Part model, mm, in its own coordinate system. Face numbers are marked on the shaded views. A direction names the side the tool comes from. Give positions to 0.01 mm unless a question says otherwise; leave off trailing zeros. Write each loop counter-clockwise with the first axis right and the second up, starting at its lowest first coordinate (ties: lowest second). Pieces come first, ordered by that corner, then holes. Notation, with made-up numbers: (66, 20.5) - (116, 20.5) arc R16 ccw to (116, 47.5) - close; hole circle Ø7 at (59.5, -25.75). An arc over 180 degrees is marked (long way). Answer in a Markdown table with one row per item. Add a question column.
1. Band-saw the part on C-C on y = -55.88. Write the cut outline in (x, z), plus the area to 3 significant figures.
2. Band-saw the part on A-A on x = 0. Write the cut outline in (y, z).
3. Which spindle directions (+Z, -Z, +X, -X, +Y, -Y) get a long thin tool onto all of the face, cutting with end or side? Do the marked faces 4, 5 and 6. Say none if no direction does.
4. Band-saw the part on B-B on z = 2. Write the cut outline in (x, y).
5. Band-saw the part on D-D on z = 33.5. Write the cut outline in (x, y), plus the area to 3 significant figures.
6. Pull direction X, two halves, no side cores. Call the marked faces 1, 2 and 3: released by +X, released by -X, zero draft, split by the parting line, or undercut.
7. Drop flat-ended pins along their axis: pin 1 Ø2.5 at (x, z) = (0, 9.5) entering from -Y; pin 2 Ø8.5 at (x, z) = (10.5, 40.5) entering from -Y; pin 3 Ø12 at (x, y) = (1.5, 35.5) entering from +Z. Give the stop position or say it passes through.
8. Probe line 1 along Y through (x, z) = (0, -7); line 2 along Y through (x, z) = (0, -3.5); line 3 along X through (y, z) = (-83.5, 12). List the from-to ranges inside material, lowest first.
```python
from build123d import *

# Parameters (mm, degrees)
F0_R           = 10.16
F1_DEPTH       = 38.1
F3_START       = 7.62
F3_DEPTH       = 27.941
F4_D           = 15.24
F4_CBORE_D     = 40.64
F4_CBORE_DEPTH = 10.16
F2_W           = 5.08
F2_H           = 76.2
F5_DEPTH       = 10.16
F6_R           = 10.16


with BuildPart() as f1:
    # F0 (on Right) → F1 (new body, symmetric)
    with BuildSketch(Plane.YZ):
        Polygon((-17.78, 15.24), (-93.98, 15.24), (-93.98, -20.32), (17.78, -20.32), (53.34, 15.24), (53.34, 50.8), (17.78, 50.8), align=None)
        Circle(F0_R, mode=Mode.SUBTRACT)
    extrude(amount=F1_DEPTH, both=True)

    # F2 (on face) → F3 (cut)
    with BuildSketch(Plane.XY.offset(15.24).offset(F3_START)):
        with BuildLine():
            Line((22.86, 43.18), (-22.86, 43.18))
            ThreePointArc((-22.86, 43.18), (-30.48, 35.56), (-22.86, 27.94))
            Line((-22.86, 27.94), (22.86, 27.94))
            ThreePointArc((22.86, 27.94), (30.48, 35.56), (22.86, 43.18))
        make_face()
    extrude(amount=F3_DEPTH, mode=Mode.SUBTRACT)

    # F4 (through all)
    with Locations(Plane.XY.offset(15.24)):
        with Locations((0, -55.88)):
            CounterBoreHole(F4_D / 2, F4_CBORE_D / 2, F4_CBORE_DEPTH)

    # F2 (on face) → F5 (cut)
    with BuildSketch(Plane.XY.offset(15.24)):
        with Locations((0, -55.88)):
            Rectangle(F2_W, F2_H)
    extrude(amount=-F5_DEPTH, mode=Mode.SUBTRACT)

    # F6
    f6_edges = [f1.edges().sort_by_distance(p)[0] for p in [
        (38.1, -93.98, -2.54),
        (-38.1, -93.98, -2.54),
        (38.1, 53.34, 33.02),
        (-38.1, 53.34, 33.02),
    ]]
    fillet(f6_edges, radius=F6_R)


solid = f1.part
```
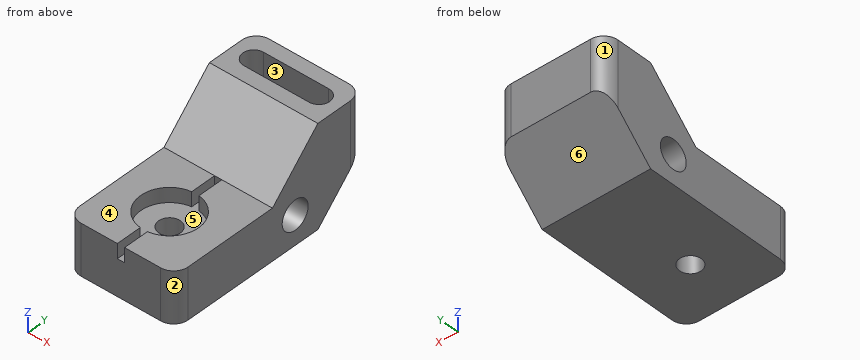
Values:
| question | item | result |
|---|---|---|
| 1 | outline | (-38.1, -20.32) - (-7.62, -20.32) - (-7.62, 5.08) - (-20.32, 5.08) - (-20.32, 15.24) - (-38.1, 15.24) - close; (7.62, -20.32) - (38.1, -20.32) - (38.1, 15.24) - (20.32, 15.24) - (20.32, 5.08) - (7.62, 5.08) - close |
| 1 | area | 1,910 mm² |
| 2 | outline | (-93.98, -20.32) - (-63.5, -20.32) - (-63.5, 5.08) - (-93.98, 5.08) - close; (-48.26, -20.32) - (17.78, -20.32) - (53.34, 15.24) - (53.34, 50.8) - (43.18, 50.8) - (43.18, 22.86) - (27.94, 22.86) - (27.94, 50.8) - (17.78, 50.8) - (-17.78, 15.24) - (-17.78, 5.08) - (-48.26, 5.08) - close; hole circle Ø20.32 at (0, 0) |
| 3 | face 4 | +Z, +X, -X, -Y |
| 3 | face 5 | +Z |
| 3 | face 6 | -Z, +X, -X, +Y |
| 4 | outline | (-38.1, -83.82) arc R10.16 ccw to (-27.94, -93.98) - (27.94, -93.98) arc R10.16 ccw to (38.1, -83.82) - (38.1, -9.96) - (-38.1, -9.96) - close; (-38.1, 9.96) - (38.1, 9.96) - (38.1, 40.1) - (-38.1, 40.1) - close; hole circle Ø15.24 at (0, -55.88) |
| 5 | outline | (-38.1, 0.48) - (38.1, 0.48) - (38.1, 43.18) arc R10.16 ccw to (27.94, 53.34) - (-27.94, 53.34) arc R10.16 ccw to (-38.1, 43.18) - close; hole (-22.86, 27.94) - (22.86, 27.94) arc R7.62 ccw to (22.86, 43.18) - (-22.86, 43.18) arc R7.62 ccw to start |
| 5 | area | 3,100 mm² |
| 6 | face 1 | released by -X |
| 6 | face 2 | released by +X |
| 6 | face 3 | undercut |
| 7 | pin 1 | stops at y = -17.78 |
| 7 | pin 2 | stops at y = 3.23 |
| 7 | pin 3 | stops at z = 22.86 |
| 8 | line 1 | y = -93.98 to -63.5, -48.26 to -7.36, 7.36 to 31.1 |
| 8 | line 2 | y = -93.98 to -63.5, -48.26 to -9.54, 9.54 to 34.6 |
| 8 | line 3 | x = -38.1 to -2.54, 2.54 to 38.1 |
